```python
from build123d import *

# Parameters (mm, degrees)
SKETCH_1_R                      = 59
SKETCH_1_R_2                    = 30
EXTRUDE_1_DEPTH                 = 8
SKETCH_2_R                      = 40
SKETCH_2_R_2                    = 35
EXTRUDE_2_DEPTH                 = 5
CUT_EXTRUDE_1_REACH             = 85.821
SKETCH_3_R                      = 4.5
CUT_EXTRUDE_1_DIRECTION_2_DEPTH = 84.821238359


with BuildPart() as part:
    # 草图1 → 凸台-拉伸1 (new body)
    with BuildSketch(Plane.XY):
        Circle(SKETCH_1_R)
        Circle(SKETCH_1_R_2, mode=Mode.SUBTRACT)
    extrude(amount=EXTRUDE_1_DEPTH)

    # 草图2 → 凸台-拉伸2 (add)
    with BuildSketch(Plane.XY.offset(8)):
        Circle(SKETCH_2_R)
        Circle(SKETCH_2_R_2, mode=Mode.SUBTRACT)
    extrude(amount=EXTRUDE_2_DEPTH)

    # 草图3 → 切除-拉伸1 (cut, up to next)
    with BuildSketch(Plane.XY.offset(8), mode=Mode.PRIVATE) as cut_extrude_1_sk1:
        with Locations((25, 43.301270189)):
            Circle(SKETCH_3_R)
    cut_extrude_1_tool1 = extrude(cut_extrude_1_sk1.sketch, amount=-CUT_EXTRUDE_1_REACH, mode=Mode.PRIVATE) & part.part
    # 草图3 → 切除-拉伸1 (cut, up to next)
    with BuildSketch(Plane.XY.offset(8), mode=Mode.PRIVATE) as cut_extrude_1_sk2:
        with Locations((50, 0)):
            Circle(SKETCH_3_R)
    cut_extrude_1_tool2 = extrude(cut_extrude_1_sk2.sketch, amount=-CUT_EXTRUDE_1_REACH, mode=Mode.PRIVATE) & part.part
    # 草图3 → 切除-拉伸1 (cut, up to next)
    with BuildSketch(Plane.XY.offset(8), mode=Mode.PRIVATE) as cut_extrude_1_sk3:
        with Locations((25, -43.301270189)):
            Circle(SKETCH_3_R)
    cut_extrude_1_tool3 = extrude(cut_extrude_1_sk3.sketch, amount=-CUT_EXTRUDE_1_REACH, mode=Mode.PRIVATE) & part.part
    # 草图3 → 切除-拉伸1 (cut, up to next)
    with BuildSketch(Plane.XY.offset(8), mode=Mode.PRIVATE) as cut_extrude_1_sk4:
        with Locations((-25, -43.301270189)):
            Circle(SKETCH_3_R)
    cut_extrude_1_tool4 = extrude(cut_extrude_1_sk4.sketch, amount=-CUT_EXTRUDE_1_REACH, mode=Mode.PRIVATE) & part.part
    # 草图3 → 切除-拉伸1 (cut, up to next)
    with BuildSketch(Plane.XY.offset(8), mode=Mode.PRIVATE) as cut_extrude_1_sk5:
        with Locations((-50, 0)):
            Circle(SKETCH_3_R)
    cut_extrude_1_tool5 = extrude(cut_extrude_1_sk5.sketch, amount=-CUT_EXTRUDE_1_REACH, mode=Mode.PRIVATE) & part.part
    # 草图3 → 切除-拉伸1 (cut, up to next)
    with BuildSketch(Plane.XY.offset(8), mode=Mode.PRIVATE) as cut_extrude_1_sk6:
        with Locations((-25, 43.301270189)):
            Circle(SKETCH_3_R)
    cut_extrude_1_tool6 = extrude(cut_extrude_1_sk6.sketch, amount=-CUT_EXTRUDE_1_REACH, mode=Mode.PRIVATE) & part.part
    add(cut_extrude_1_tool1.solids().sort_by_distance((25, 43.30127, 8))[0], mode=Mode.SUBTRACT)
    add(cut_extrude_1_tool2.solids().sort_by_distance((50, 0, 8))[0], mode=Mode.SUBTRACT)
    add(cut_extrude_1_tool3.solids().sort_by_distance((25, -43.30127, 8))[0], mode=Mode.SUBTRACT)
    add(cut_extrude_1_tool4.solids().sort_by_distance((-25, -43.30127, 8))[0], mode=Mode.SUBTRACT)
    add(cut_extrude_1_tool5.solids().sort_by_distance((-50, 0, 8))[0], mode=Mode.SUBTRACT)
    add(cut_extrude_1_tool6.solids().sort_by_distance((-25, 43.30127, 8))[0], mode=Mode.SUBTRACT)

    # 草图3 → 切除-拉伸1 direction 2 (cut)
    with BuildSketch(Plane.XY.offset(8)):
        with Locations((25, 43.301270189)):
            Circle(SKETCH_3_R)
        with Locations((50, 0)):
            Circle(SKETCH_3_R)
        with Locations((25, -43.301270189)):
            Circle(SKETCH_3_R)
        with Locations((-25, -43.301270189)):
            Circle(SKETCH_3_R)
        with Locations((-50, 0)):
            Circle(SKETCH_3_R)
        with Locations((-25, 43.301270189)):
            Circle(SKETCH_3_R)
    extrude(amount=CUT_EXTRUDE_1_DIRECTION_2_DEPTH, mode=Mode.SUBTRACT)


solid = part.part
```
Verification items for the finished model (mm, model axes). A direction names the side the tool comes from. Coordinates: 2 decimals unless noted, no trailing zeros. Loops run counter-clockwise (first coordinate to the right, second up) from the corner with the lowest first, then second, coordinate; pieces in that order, holes last. Notation, with made-up numbers: (-21, 5.5) - (19, 5.5) arc R20 ccw to (19, 22.5) - close; hole circle Ø8 at (31.25, 68). An arc over 180 degrees is marked (long way). Put each result on its own line as item: value.
Item 1: Set-up check for faces 1 (the face through (-45.708, 1.352, 4.056)), 2 (the face through (12, -39, 8)): record each of +Z, -Z, +X, -X, +Y, -Y from which the full face is reachable in a straight line by a thin tool's end or side.
Conclusion:
face 1: +Z, -Z
face 2: +Z
Item 2: Gauge pin test, flat ends, axial feed: pin 1 Ø11.5 at (x, y) = (25, 43.3) entering from +Z; pin 2 Ø1 at (y, z) = (-27.5, 5.5) entering from -X; pin 3 Ø11.5 at (x, y) = (50, 0) entering from -Z; pin 4 Ø2 at (y, z) = (-25, 9.5) entering from +X. Record the tip position at first contact, or that the pin passes through.
Conclusion:
pin 1: stops at z = 8
pin 2: stops at x = -52.46
pin 3: stops at z = 0
pin 4: stops at x = 32
Item 3: Section check D-D (z = 5.5). Enter the section's corners in (x, y).
Conclusion:
outline: circle Ø118 at (0, 0); hole circle Ø9 at (-50, 0); hole circle Ø60 at (0, 0); hole circle Ø9 at (-25, -43.3); hole circle Ø9 at (-25, 43.3); hole circle Ø9 at (25, -43.3); hole circle Ø9 at (25, 43.3); hole circle Ø9 at (50, 0)
Item 4: Section check A-A (x = 0). Enter the section's corners in (y, z).
Conclusion:
outline: (-59, 0) - (-30, 0) - (-30, 8) - (-35, 8) - (-35, 13) - (-40, 13) - (-40, 8) - (-59, 8) - close; (30, 0) - (59, 0) - (59, 8) - (40, 8) - (40, 13) - (35, 13) - (35, 8) - (30, 8) - close
Item 5: Scan lines: line 1 along Y through (x, z) = (0, 11.65); line 2 along Y through (x, z) = (-25, 2); line 3 along X through (y, z) = (-45.5, 3.25). Record each from-to range of solid material in increasing order.
Conclusion:
line 1: y = -40 to -35, 35 to 40
line 2: y = -53.44 to -47.8, -38.8 to -16.58, 16.58 to 38.8, 47.8 to 53.44
line 3: x = -37.56 to -28.93, -21.07 to 21.07, 28.93 to 37.56
Item 6: Draft check along Y on faces 3 (the face through (-0.2, -35.4, 13)), 4 (the face through (26, 16, 8)), 5 (the face through (-8.67, -39.05, 10.46)). Enter one of: pulls with the +Y half, pulls with the -Y half, needs draft (parallel to the pull), parting line crosses it, or undercut.
Conclusion:
face 3: needs draft
face 4: undercut
face 5: parting line crosses it
Item 7: Section check B-B (y = 0). Enter the section's corners in (x, z), then the cut area to 3 significant figures.
Conclusion:
outline: (-59, 0) - (-54.5, 0) - (-54.5, 8) - (-59, 8) - close; (-45.5, 0) - (-30, 0) - (-30, 8) - (-35, 8) - (-35, 13) - (-40, 13) - (-40, 8) - (-45.5, 8) - close; (30, 0) - (45.5, 0) - (45.5, 8) - (40, 8) - (40, 13) - (35, 13) - (35, 8) - (30, 8) - close; (54.5, 0) - (59, 0) - (59, 8) - (54.5, 8) - close
area: 370 mm2
Item 8: Section check C-C (x = -25). Enter the section's corners in (y, z).
Conclusion:
outline: (-53.44, 0) - (-47.8, 0) - (-47.8, 8) - (-53.44, 8) - close; (-38.8, 0) - (-16.58, 0) - (-16.58, 8) - (-24.49, 8) - (-24.49, 13) - (-31.22, 13) - (-31.22, 8) - (-38.8, 8) - close; (16.58, 0) - (38.8, 0) - (38.8, 8) - (31.22, 8) - (31.22, 13) - (24.49, 13) - (24.49, 8) - (16.58, 8) - close; (47.8, 0) - (53.44, 0) - (53.44, 8) - (47.8, 8) - close
